Check sheet for the modelled part. Datum: model origin and axes. Units: mm. A direction names the side the tool comes from. Round coordinates to 2 decimals unless told otherwise and drop trailing zeros.
from build123d import *

# Parameters (mm, degrees)
SKETCH1_W           = 100
SKETCH1_H           = 100
BOSS_EXTRUDE2_DEPTH = 35
FILLET3_R           = 10
FILLET4_R           = 5
SKETCH2_R           = 7.5
CUT_EXTRUDE1_DEPTH  = 1
CUT_EXTRUDE2_DEPTH  = 1


with BuildPart() as part:
    # Sketch1 → Boss-Extrude2 (new body)
    with BuildSketch(Plane.XY):
        with Locations((-7.378614961, -23.844584937)):
            Rectangle(SKETCH1_W, SKETCH1_H)
    extrude(amount=BOSS_EXTRUDE2_DEPTH)

    # Fillet3
    fillet3_edges = [part.edges().sort_by_distance(p)[0] for p in [
        (-57.378614961, 26.155415063, 17.5),
        (42.621385039, 26.155415063, 17.5),
        (42.621385039, -73.844584937, 17.5),
        (-57.378614961, -73.844584937, 17.5),
    ]]
    fillet(fillet3_edges, radius=FILLET3_R)

    # Fillet4
    fillet4_edges = [part.edges().sort_by_distance(p)[0] for p in [
        (42.621385039, -23.844584937, 35),
        (-7.378614961, -73.844584937, 35),
        (-57.378614961, -23.844584937, 35),
        (-7.378614961, 26.155415063, 35),
        (39.692452851, 23.226482875, 35),
        (-54.449682772, 23.226482875, 35),
        (-54.449682772, -70.915652749, 35),
        (39.692452851, -70.915652749, 35),
    ]]
    fillet(fillet4_edges, radius=FILLET4_R)

    # Sketch2 → Cut-Extrude1 (cut)
    with BuildSketch(Plane(origin=(42.621385039, 0, 0), x_dir=(0, 0, -1), z_dir=(1, 0, 0))):
        with Locations((-14.550369157, -50.784546634)):
            Circle(SKETCH2_R)
    extrude(amount=-CUT_EXTRUDE1_DEPTH, mode=Mode.SUBTRACT)

    # Sketch3 → Cut-Extrude2 (cut)
    with BuildSketch(Plane.XY.offset(35)):
        with BuildLine():
            Line((-19.273762165, -36.822061823), (-19.273762165, -26.851128879))
            ThreePointArc((-19.273762165, -26.851128879), (-16.017889756, -23.595256471), (-12.762017347, -26.851128879))
            Line((-12.762017347, -26.851128879), (-12.762017347, -36.822061823))
            ThreePointArc((-12.762017347, -36.822061823), (-16.017889756, -40.077934232), (-19.273762165, -36.822061823))
        make_face()
        with BuildLine():
            Line((-11.027771482, -29.224294891), (-11.027771482, -19.253361947))
            ThreePointArc((-11.027771482, -19.253361947), (-7.771899073, -15.997489538), (-4.516026664, -19.253361947))
            Line((-4.516026664, -19.253361947), (-4.516026664, -29.224294891))
            ThreePointArc((-4.516026664, -29.224294891), (-7.771899073, -32.4801673), (-11.027771482, -29.224294891))
        make_face()
        with BuildLine():
            Line((-2.681741214, -21.311514936), (-2.681741214, -11.340581993))
            ThreePointArc((-2.681741214, -11.340581993), (0.574131194, -8.084709584), (3.830003603, -11.340581993))
            Line((3.830003603, -11.340581993), (3.830003603, -21.311514936))
            ThreePointArc((3.830003603, -21.311514936), (0.574131194, -24.567387345), (-2.681741214, -21.311514936))
        make_face()
    extrude(amount=-CUT_EXTRUDE2_DEPTH, mode=Mode.SUBTRACT)


solid = part.part
1) Draft check along X on faces 1 (the face through (0.503, -8.085, 34.507)), 2 (the face through (1, -16, 34)), 3 (the face through (-8, -73.845, 15)), 4 (the face through (-57.379, -24, 15)). Enter one of: pulls with the +X half, pulls with the -X half, needs draft (parallel to the pull), parting line crosses it, or undercut.
2) Gauge pin test, flat ends, axial feed: pin 1 (0.8 mm diameter, centred on y = -22, z = 34.5, fed in from -X); pin 2 (1.1 mm diameter, centred on y = -23, z = 34.5, fed in from +X); pin 3 (0.8 mm diameter, centred on y = -16.5, z = 34.5, fed in from +X). Record the tip position at first contact, or that the pin passes through.
3) Scan lines: line 1 (Z direction, x = -5, y = -21); line 2 (Y direction, x = 0, z = 30.5); line 3 (Y direction, x = 37, z = 20.5) (3 decimals). Record each from-to range of solid material in increasing order.
4) Set-up check for faces 5 (the face through (-16.089, -23.596, 34.507)), 6 (the face through (42.13, -55.35, 20.5)), 7 (the face through (-8, -23, 0)): record each of +Z, -Z, +X, -X, +Y, -Y from which the full face is reachable in a straight line by a thin tool's end or side.
Values found:
1. face 1: undercut
1. face 2: undercut
1. face 3: needs draft
1. face 4: pulls with the -X half
2. pin 1: stops at x = -55.24
2. pin 2: stops at x = 40.69
2. pin 3: stops at x = 40.48
3. line 1: z = 0 to 34
3. line 2: y = -73.82 to 26.13
3. line 3: y = -72.835 to 25.146
4. face 5: +Z
4. face 6: +X
4. face 7: -Z, +X, -X, +Y, -Y
